from build123d import *

# Parameters (mm, degrees)
BOSS_EXTRUDE1_DEPTH = 59


with BuildPart() as part:
    # Sketch1 → Boss-Extrude1 (new body)
    with BuildSketch(Plane.XY):
        with BuildLine():
            Line((141.836213574, 162.11895664), (136.686788287, 172.578726755))
            Line((136.686788287, 172.578726755), (101.422420471, 158.233899169))
            Line((101.422420471, 158.233899169), (53.008627367, 148.670680778))
            Line((53.008627367, 148.670680778), (53.008627367, 145.981025606))
            Line((53.008627367, 145.981025606), (27.307477942, 143.590221008))
            Line((27.307477942, 143.590221008), (27.307477942, 158.233899169))
            Line((27.307477942, 158.233899169), (19.307477942, 158.233899169))
            Line((19.307477942, 158.233899169), (19.307477942, 143.590221008))
            ThreePointArc((19.307477942, 143.590221008), (8.621741422, 136.172049269), (11.836213574, 123.567232502))
            ThreePointArc((11.836213574, 123.567232502), (15.367024557, 116.508815615), (12.8726305, 109.02110078))
            ThreePointArc((12.8726305, 109.02110078), (10.487522097, 97.279293257), (19.307477942, 89.169597523))
            Line((19.307477942, 89.169597523), (19.307477942, 58.363836225))
            Line((19.307477942, 58.363836225), (14.461757095, 58.363836225))
            Line((14.461757095, 58.363836225), (14.461757095, 32.578726755))
            Line((14.461757095, 32.578726755), (31.423101088, 32.578726755))
            Line((31.423101088, 32.578726755), (31.423101088, 63.242577829))
            Line((31.423101088, 63.242577829), (27.307477942, 63.242577829))
            Line((27.307477942, 63.242577829), (27.307477942, 93.887357851))
            ThreePointArc((27.307477942, 93.887357851), (29.389559507, 93.024931429), (30.251985929, 90.942849864))
            Line((30.251985929, 90.942849864), (30.251985929, 87.578726755))
            Line((30.251985929, 87.578726755), (73.151157521, 87.578726755))
            Line((73.151157521, 87.578726755), (73.151157521, 91.578726755))
            Line((73.151157521, 91.578726755), (73.151157521, 115.775958178))
            ThreePointArc((73.151157521, 115.775958178), (68.856721822, 123.355383827), (60.147818832, 123.567232502))
            Line((60.147818832, 123.567232502), (59.530992057, 123.567232502))
            Line((59.530992057, 123.567232502), (92.194583693, 139.647769923))
            Line((92.194583693, 139.647769923), (141.836213574, 159.840975298))
            Line((141.836213574, 159.840975298), (141.836213574, 162.11895664))
        make_face()
    extrude(amount=BOSS_EXTRUDE1_DEPTH)


solid = part.part
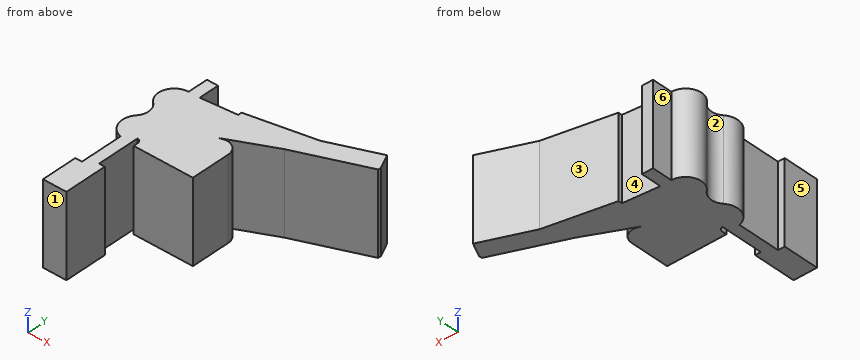
Here's how the part is built. I have some questions about the finished solid (model axes, mm). Face numbers are marked on the shaded views. A direction names the side the tool comes from. Give positions to 0.01 mm unless a question says otherwise; leave off trailing zeros. Order: outer loops, then holes, each group sorted by start corner. A loop starts at its lowest first (then second) coordinate and runs counter-clockwise, first axis right, second up. Notation, with made-up numbers: (-36.75, 68) -> (-17.75, 68) arc R35 cw to (-17.75, 105) -> close; hole circle Ø4 at (59, 76.25). An arc over 180 degrees is marked (long way). Use a Markdown table: item, result. Add a question column.
Item 1: If we mould it in two halves opening along X, with no side actions, what happens to the marked faces 1, 2 and 3? For each: pulls with the +X half, pulls with the -X half, needs draft (parallel to the pull), parting line crosses it, or undercut.
Item 2: Will these pins go through, and if not, where does the flat tip stop? pin 1 (5 mm diameter, centred on y = 102.5, z = 12, fed in from +X); pin 2 (9 mm diameter, centred on y = 81, z = 20, fed in from +X); pin 3 (0.8 mm diameter, centred on y = 147.5, z = 30, fed in from -X).
Item 3: Imagine slicing it at B-B on y = 43.5. Please give me the cut outline in (x, z), plus the area to 3 significant figures.
Item 4: Imagine slicing it at C-C on x = 21.5. Please give me the cut outline in (y, z), plus the area to 3 significant figures.
Item 5: Imagine slicing it at A-A on z = 37.5. Please give me the cut outline in (x, y).
Item 6: For the marked faces 4, 5 and 6, which set-ups out of +Z, -Z, +X, -X, +Y, -Y let a thin tool reach every point of the face, with its end or its side?
Item 7: I need wall thicknesses on line 1 (X direction, y = 73, z = 45); line 2 (X direction, y = 49.5, z = 37); line 3 (Y direction, x = 66, z = 14). Which ranges of each line are inside material? Lowest first, please.
Data:
| question | item | result |
|---|---|---|
| 1 | face 1 | needs draft |
| 1 | face 2 | pulls with the -X half |
| 1 | face 3 | undercut |
| 2 | pin 1 | stops at x = 73.15 |
| 2 | pin 2 | stops at x = 27.31 |
| 2 | pin 3 | stops at x = 19.31 |
| 3 | outline | (14.46, 0) -> (31.42, 0) -> (31.42, 59) -> (14.46, 59) -> close |
| 3 | area | 1,000 mm² |
| 4 | outline | (32.58, 0) -> (158.23, 0) -> (158.23, 59) -> (32.58, 59) -> close |
| 4 | area | 7,410 mm² |
| 5 | outline | (11.84, 123.57) arc R10.31 cw to (12.87, 109.02) arc R12.19 ccw to (19.31, 89.17) -> (19.31, 58.36) -> (14.46, 58.36) -> (14.46, 32.58) -> (31.42, 32.58) -> (31.42, 63.24) -> (27.31, 63.24) -> (27.31, 93.89) arc R2.94 cw to (30.25, 90.94) -> (30.25, 87.58) -> (73.15, 87.58) -> (73.15, 115.78) arc R8.84 ccw to (60.15, 123.57) -> (59.53, 123.57) -> (92.19, 139.65) -> (141.84, 159.84) -> (141.84, 162.12) -> (136.69, 172.58) -> (101.42, 158.23) -> (53.01, 148.67) -> (53.01, 145.98) -> (27.31, 143.59) -> (27.31, 158.23) -> (19.31, 158.23) -> (19.31, 143.59) arc R11.41 ccw to start |
| 6 | face 4 | +Z, -Z, +Y |
| 6 | face 5 | +Z, -Z, -X, -Y |
| 6 | face 6 | +Z, -Z, -X, +Y |
| 7 | line 1 | x = 19.31 to 27.31 |
| 7 | line 2 | x = 14.46 to 31.42 |
| 7 | line 3 | y = 87.58 to 124.45, 126.75 to 151.24 |
